from build123d import *

# Parameters (mm, degrees)
BOSS_EXTRUDE1_DEPTH = 10
SKETCH2_W           = 4.3
SKETCH2_H           = 5
CUT_EXTRUDE1_DEPTH  = 5.3
SKETCH3_R           = 1.368686713
SKETCH3_W           = 4
SKETCH3_H           = 0.5
CUT_EXTRUDE2_DEPTH  = 5


with BuildPart() as part:
    # Sketch1 → Boss-Extrude1 (new body)
    with BuildSketch(Plane.XY):
        Polygon((-3.415220484, 0), (4.584779516, 0), (4.584779516, 6.2), (3.274734062, 10.00055008), (-1.425265938, 10.00055008), (-3.415220484, 6.2), align=None)
    extrude(amount=BOSS_EXTRUDE1_DEPTH)

    # Sketch2 → Cut-Extrude1 (cut)
    with BuildSketch(Plane(origin=(4.584779516, 0, 0), x_dir=(0, 0, -1), z_dir=(1, 0, 0))):
        with Locations((-7.5, 3.1)):
            Rectangle(SKETCH2_W, SKETCH2_H)
        with Locations((-2.5, 3.1)):
            Rectangle(SKETCH2_W, SKETCH2_H)
    extrude(amount=-CUT_EXTRUDE1_DEPTH, mode=Mode.SUBTRACT)

    # Sketch3 → Cut-Extrude2 (cut)
    with BuildSketch(Plane(origin=(0, 10.00055008, 0), x_dir=(1, 0, 0), z_dir=(0, 1, 0))):
        with Locations((0.924734062, -2.85)):
            Circle(SKETCH3_R)
        with Locations((0.924734062, -7.15)):
            Circle(SKETCH3_R)
        with Locations((0.924734062, -5)):
            Rectangle(SKETCH3_W, SKETCH3_H)
    extrude(amount=-CUT_EXTRUDE2_DEPTH, mode=Mode.SUBTRACT)


solid = part.part
Build history of the part. All positions in model axes, mm. A direction names the side the tool comes from. Coordinates: 2 decimals unless noted, no trailing zeros. Order: outer loops, then holes, each group sorted by start corner. A loop starts at its lowest first (then second) coordinate and runs counter-clockwise, first axis right, second up. Notation, with made-up numbers: (7.25, 31) - (25.25, 31) arc R27 cw to (25.25, 59) - close; hole circle Ø1 at (3, -1). An arc over 180 degrees is marked (long way). Write item = value, one per line. Start each with the question number.
1) Saw through at B-B on y = 5.25. Write the cut outline in (x, z), then the cut area to 3 significant figures.
2) 3-axis set-ups, long thin cutter, end or side, ignore diameter. For faces 4 (the face through (2, 0.6, 3)), 5 (the face through (-3.415, 3, 5)), 6 (the face through (1, 8, 5.25)): which of +Z, -Z, +X, -X, +Y, -Y reach the whole face in a straight line?
3) Saw through at A-A on z = 7.15. Write the cut outline in (x, y), then the cut area to 3 significant figures.
4) Saw through at D-D on z = 5. Write the cut outline in (x, y).
5) Two-plate mould, pull along X, no slides. Class faces 1 (the face through (0.628, 7.831, 4.186)), 2 (the face through (-0.715, 3, 8)), 3 (the face through (2, 3, 5.35)): pulls with the +X half, pulls with the -X half, needs draft (parallel to the pull), parting line crosses it, or undercut.
6) Wall check: line 1 along Z through (x, y) = (3.25, 4.25); line 2 along Z through (x, y) = (2.75, 8); line 3 along Z through (x, y) = (1.5, 8). Give the ranges that are in metal, low to high. Write a range as from..to.
7) Saw through at C-C on y = 6.75. Write the cut outline in (x, z).
8) Flat gauge pin, fed straight in: pin 1 Ø1.6 at (x, z) = (0.92, 2.85) entering from +Y. Where does the tip first touch, or does it go through?
From the geometry:
q1.outline = (-3.42, 0) - (4.58, 0) - (4.58, 0.35) - (-0.72, 0.35) - (-0.72, 4.65) - (4.58, 4.65) - (4.58, 5.35) - (-0.72, 5.35) - (-0.72, 9.65) - (4.58, 9.65) - (4.58, 10) - (-3.42, 10) - close; hole (-1.08, 4.75) - (2.92, 4.75) - (2.92, 5.25) - (-1.08, 5.25) - close
q1.area = 32.4 mm^2
q2.face_4 = +X
q2.face_5 = +Z, -Z, -X, +Y, -Y
q2.face_6 = +Y
q3.outline = (-3.42, 0) - (4.58, 0) - (4.58, 0.6) - (-0.72, 0.6) - (-0.72, 5.6) - (-0.44, 5.6) - (-0.44, 10) - (-1.43, 10) - (-3.42, 6.2) - close; (2.29, 5.6) - (4.58, 5.6) - (4.58, 6.2) - (3.27, 10) - (2.29, 10) - close
q3.area = 35.2 mm^2
q4.outline = (-3.42, 0) - (4.58, 0) - (4.58, 6.2) - (3.27, 10) - (2.92, 10) - (2.92, 5) - (-1.08, 5) - (-1.08, 10) - (-1.43, 10) - (-3.42, 6.2) - close
q5.face_1 = undercut
q5.face_2 = pulls with the +X half
q5.face_3 = needs draft
q6.line_1 = 0..0.35, 4.65..5.35, 9.65..10
q6.line_2 = 0..4.75, 5.25..10
q6.line_3 = 0..1.61, 4.09..4.75, 5.25..5.91, 8.39..10
q7.outline = (-3.13, 0) - (4.4, 0) - (4.4, 10) - (-3.13, 10) - close; hole (-1.08, 4.75) - (2.92, 4.75) - (2.92, 5.25) - (-1.08, 5.25) - close; hole circle Ø2.74 at (0.92, 2.85); hole circle Ø2.74 at (0.92, 7.15)
q8.pin_1 = 0.6
